The listing builds one solid part. Answer for the finished solid, in the listing's coordinates (mm). Face numbers are marked on the shaded views. A direction names the side the tool comes from. Round coordinates to 2 decimals unless told otherwise and drop trailing zeros. Loops run counter-clockwise (first coordinate to the right, second up) from the corner with the lowest first, then second, coordinate; pieces in that order, holes last. Notation, with made-up numbers: M 4,21.5 L 59,21.5 A13 ccw 59,43.5 Z; hole C -18.5,-6 d10. An arc over 180 degrees is marked long. Put each result on its own line as item: value. Start each with the question number.
(1) Determine the mould class of the marked faces 3, 4 and 5 for opening direction Z: released by +Z, released by -Z, zero draft, split by the parting line, or undercut.
(2) Section A-A, the plane z = 0 is taken. Determine the outline of the cut face in (x, y) (3 decimals).
(3) Flat-ended cylindrical pins translate along their axes: P1, Ø1, axis at y = 28.5, z = -7, coming from the -X side; P2, Ø1.5, axis at x = -6, z = 5, coming from the +Y side; P3, Ø8, axis at y = 16, z = -7, coming from the -X side. Find the tip coordinate at first contact, or state that the pin passes through.
(4) Straight lines are drawn through the part: line 1 (Z direction, x = 0, y = 49) (3 decimals); line 2 (Y direction, x = -2.5, z = -4.25); line 3 (Z direction, x = -7.5, y = 49). For each, find the intervals that lie inside material, in ascending order.
(5) Section D-D, the plane x = 6 is taken. Determine the outline of the cut face in (y, z), then the cut area to 3 significant figures.
(6) Which of the six approach directions +Z, -Z, +X, -X, +Y, -Y give full straight-line access (tool end or side, diameter ignored) to the marked faces 1 and 2?
(7) Section B-B, the plane x = 0 is taken. Determine the outline of the cut face in (y, z) (3 decimals), then the cut area to 3 significant figures.
```python
from build123d import *

# Parameters (mm, degrees)
F4_R      = 9.525
F6_DEPTH  = 50.8
F5_R      = 0.7691273294
F7_DEPTH  = 50.8
F8_R      = 0.51181
F10_DEPTH = 9.525
F9_R      = 3.175
F11_DEPTH = 63.5
F12_R     = 1.18745
F13_DEPTH = 69.85


with BuildPart() as f6:
    # F4 (on Front) → F6 (new body)
    with BuildSketch(Plane.XZ):
        Circle(F4_R)
    extrude(amount=-F6_DEPTH)

    # F5 (on Front) → F7 (join)
    with BuildSketch(Plane.XZ):
        with Locations((-2.815608135, 9.0993393073)):
            Circle(F5_R)
        with Locations((4.4432689231, 8.4251401339)):
            Circle(F5_R)
        with Locations((9.0993393073, 2.815608135)):
            Circle(F5_R)
        with Locations((8.4251401339, -4.4432689231)):
            Circle(F5_R)
        with Locations((2.815608135, -9.0993393073)):
            Circle(F5_R)
        with Locations((-4.4432689231, -8.4251401339)):
            Circle(F5_R)
        with Locations((-9.0993393073, -2.815608135)):
            Circle(F5_R)
        with Locations((-8.4251401339, 4.4432689231)):
            Circle(F5_R)
    extrude(amount=-F7_DEPTH)

    # F8 (on Front) → F10 (cut)
    with BuildSketch(Plane.XZ):
        Circle(F8_R)
    extrude(amount=-F10_DEPTH, mode=Mode.SUBTRACT)

    # F9 (on Front) → F11 (join)
    with BuildSketch(Plane.XZ):
        Circle(F9_R)
    extrude(amount=-F11_DEPTH)

    # F12 (on Front) → F13 (cut)
    with BuildSketch(Plane.XZ):
        Circle(F12_R)
    extrude(amount=-F13_DEPTH, mode=Mode.SUBTRACT)


solid = f6.part
```
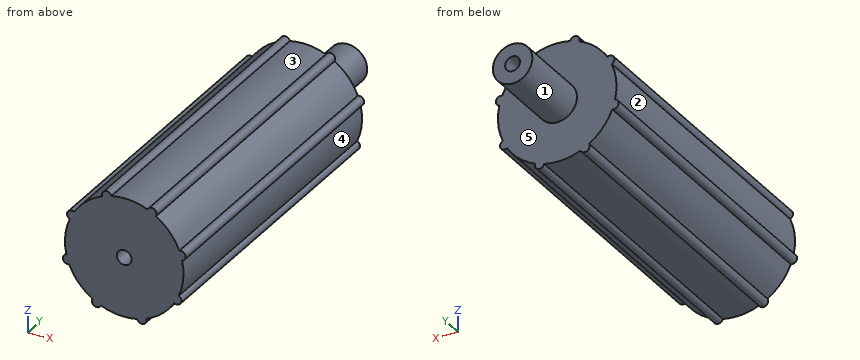
Recorded:
1. face 3: released by +Z
1. face 4: undercut
1. face 5: zero draft
2. outline: M -9.525,0 L -1.187,0 L -1.187,63.5 L -3.175,63.5 L -3.175,50.8 L -9.525,50.8 Z; M 1.187,0 L 9.525,0 L 9.525,50.8 L 3.175,50.8 L 3.175,63.5 L 1.187,63.5 Z
3. P1: stops at x = -6.96
3. P2: stops at y = 50.8
3. P3: stops at x = -9.85
4. line 1: z = -9.525 to -1.187, 1.187 to 9.525
4. line 2: y = 0 to 50.8
4. line 3: z = -5.87 to 5.87
5. outline: M 0,-7.4 L 50.8,-7.4 L 50.8,7.4 L 0,7.4 Z
5. area: 752 mm²
6. face 1: +Y
6. face 2: -X, +Y, -Y
7. outline: M 0,-9.525 L 50.8,-9.525 L 50.8,-3.175 L 63.5,-3.175 L 63.5,-1.187 L 0,-1.187 Z; M 0,1.187 L 63.5,1.187 L 63.5,3.175 L 50.8,3.175 L 50.8,9.525 L 0,9.525 Z
7. area: 898 mm²
